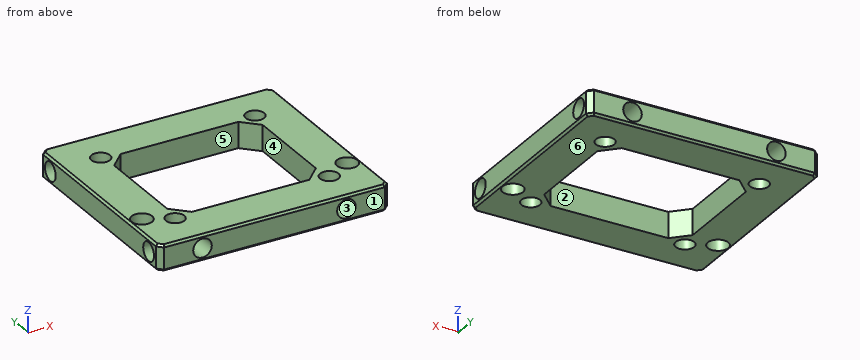
from build123d import *

# Parameters (mm, degrees)
SKETCH2_W               = 44.8
SKETCH2_H               = 39.8
SKETCH2_W_2             = 28.8
SKETCH2_H_2             = 23.8
BOSS_EXTRUDE1_DEPTH     = 5
CHAMFER1_SIZE           = 1
CHAMFER2_SIZE           = 3
SKETCH3_R               = 1.8
CUT_EXTRUDE1_DEPTH      = 6
SKETCH4_R               = 1.8
CUT_EXTRUDE2_DEPTH      = 5
SKETCH5_R               = 1.8
CUT_EXTRUDE3_DEPTH      = 5
MIRROR2_COPY_1_SKETCH_R = 1.8
MIRROR2_COPY_1_DEPTH    = 6
MIRROR2_COPY_2_SKETCH_R = 1.8
MIRROR2_COPY_2_DEPTH    = 5
MIRROR2_COPY_3_SKETCH_R = 1.8
MIRROR2_COPY_3_DEPTH    = 5
SKETCH6_R               = 2
CUT_EXTRUDE4_DEPTH      = 6
CHAMFER3_SIZE           = 0.4


with BuildPart() as part:
    # Sketch2 → Boss-Extrude1 (new body)
    with BuildSketch(Plane.XY):
        Rectangle(SKETCH2_W, SKETCH2_H)
        Rectangle(SKETCH2_W_2, SKETCH2_H_2, mode=Mode.SUBTRACT)
    extrude(amount=BOSS_EXTRUDE1_DEPTH)

    # Chamfer1
    chamfer1_edges = [part.edges().sort_by_distance(p)[0] for p in [
        (-22.4, 19.9, 2.5),
        (22.4, 19.9, 2.5),
        (22.4, -19.9, 2.5),
        (-22.4, -19.9, 2.5),
    ]]
    chamfer(chamfer1_edges, length=CHAMFER1_SIZE)

    # Chamfer2
    chamfer2_edges = [part.edges().sort_by_distance(p)[0] for p in [
        (-14.4, 11.9, 2.5),
        (-14.4, -11.9, 2.5),
        (14.4, -11.9, 2.5),
        (14.4, 11.9, 2.5),
    ]]
    chamfer(chamfer2_edges, length=CHAMFER2_SIZE)

    # Sketch3 → Cut-Extrude1 (cut, through all)
    with BuildSketch(Plane.XY.offset(5)):
        with Locations((14.95, 12.45)):
            Circle(SKETCH3_R)
    cut_extrude1 = extrude(amount=-CUT_EXTRUDE1_DEPTH, mode=Mode.SUBTRACT)

    # Sketch4 → Cut-Extrude2 (cut)
    with BuildSketch(Plane(origin=(0, 19.9, 0), x_dir=(1, 0, 0), z_dir=(0, 1, 0))):
        with Locations((13.95, -2.5)):
            Circle(SKETCH4_R)
    cut_extrude2 = extrude(amount=-CUT_EXTRUDE2_DEPTH, mode=Mode.SUBTRACT)

    # Sketch5 → Cut-Extrude3 (cut)
    with BuildSketch(Plane(origin=(22.4, 0, 0), x_dir=(0, 0, -1), z_dir=(1, 0, 0))):
        with Locations((-2.5, 16.45)):
            Circle(SKETCH5_R)
    cut_extrude3 = extrude(amount=-CUT_EXTRUDE3_DEPTH, mode=Mode.SUBTRACT)

    # Mirror1: Cut-Extrude1, Cut-Extrude2, Cut-Extrude3 across plane
    add(cut_extrude1.mirror(Plane.ZX), mode=Mode.SUBTRACT)
    add(cut_extrude2.mirror(Plane.ZX), mode=Mode.SUBTRACT)
    add(cut_extrude3.mirror(Plane.ZX), mode=Mode.SUBTRACT)

    # Mirror2: Cut-Extrude1, Cut-Extrude2, Cut-Extrude3 across plane
    add(cut_extrude1.mirror(Plane(origin=(0, 0, 0), x_dir=(0, 0, 1), z_dir=(1, 0, 0))), mode=Mode.SUBTRACT)
    add(cut_extrude2.mirror(Plane(origin=(0, 0, 0), x_dir=(0, 0, 1), z_dir=(1, 0, 0))), mode=Mode.SUBTRACT)
    add(cut_extrude3.mirror(Plane(origin=(0, 0, 0), x_dir=(0, 0, 1), z_dir=(1, 0, 0))), mode=Mode.SUBTRACT)

    # Mirror2 copy 1 sketch → Mirror2 copy 1 (cut, through all)
    with BuildSketch(Plane(origin=(0, 0, 5), x_dir=(-1, 0, 0), z_dir=(0, 0, 1))):
        with Locations((14.95, 12.45)):
            Circle(MIRROR2_COPY_1_SKETCH_R)
    extrude(amount=-MIRROR2_COPY_1_DEPTH, mode=Mode.SUBTRACT)

    # Mirror2 copy 2 sketch → Mirror2 copy 2 (cut)
    with BuildSketch(Plane(origin=(0, -19.9, 0), x_dir=(-1, 0, 0), z_dir=(0, -1, 0))):
        with Locations((13.95, -2.5)):
            Circle(MIRROR2_COPY_2_SKETCH_R)
    extrude(amount=-MIRROR2_COPY_2_DEPTH, mode=Mode.SUBTRACT)

    # Mirror2 copy 3 sketch → Mirror2 copy 3 (cut)
    with BuildSketch(Plane(origin=(-22.4, 0, 0), x_dir=(0, 0, -1), z_dir=(-1, 0, 0))):
        with Locations((-2.5, 16.45)):
            Circle(MIRROR2_COPY_3_SKETCH_R)
    extrude(amount=-MIRROR2_COPY_3_DEPTH, mode=Mode.SUBTRACT)

    # Sketch6 → Cut-Extrude4 (cut, through all)
    with BuildSketch(Plane.XY.offset(5)):
        with Locations((19.9, -9.9)):
            Circle(SKETCH6_R)
        with Locations((-19.9, -9.9)):
            Circle(SKETCH6_R)
    extrude(amount=-CUT_EXTRUDE4_DEPTH, mode=Mode.SUBTRACT)

    # Chamfer3
    chamfer3_edges = [part.edges().sort_by_distance(p)[0] for p in [
        (0, -19.9, 0),
        (0, -19.9, 5),
        (-22.4, 0, 0),
        (0, 19.9, 0),
        (22.4, 0, 0),
        (-21.9, 19.4, 0),
        (21.9, 19.4, 0),
        (21.9, -19.4, 0),
        (-21.9, -19.4, 0),
        (-22.4, 0, 5),
        (22.4, 0, 5),
        (0, 19.9, 5),
        (-21.9, 19.4, 5),
        (21.9, 19.4, 5),
        (21.9, -19.4, 5),
        (-21.9, -19.4, 5),
    ]]
    chamfer(chamfer3_edges, length=CHAMFER3_SIZE)


solid = part.part
Geometry check sheet. Reference: the model listing, model coordinates, mm. Face numbers are marked on the shaded views. A direction names the side the tool comes from. Give positions to 0.01 mm unless a question says otherwise; leave off trailing zeros. Write each loop counter-clockwise with the first axis right and the second up, starting at its lowest first coordinate (ties: lowest second). Pieces come first, ordered by that corner, then holes. Notation, with made-up numbers: (-39, 2.25) - (-15, 2.25) arc R8 ccw to (-15, 13.25) - close; hole circle Ø4 at (-16.75, 5.5). An arc over 180 degrees is marked (long way). Put each result on its own line as item: value.
1. Set-up check for the marked faces 5 and 6: record each of +Z, -Z, +X, -X, +Y, -Y from which the full face is reachable in a straight line by a thin tool's end or side.
Ans:
face 5: +Z, -Z
face 6: -Z, +X, -X, +Y, -Y
2. Sectioned sample at C-C, the plane x = -2.5. Enter the section's corners in (y, z).
Ans:
outline: (-19.9, 0.4) - (-19.5, 0) - (-11.9, 0) - (-11.9, 5) - (-19.5, 5) - (-19.9, 4.6) - close; (11.9, 0) - (19.5, 0) - (19.9, 0.4) - (19.9, 4.6) - (19.5, 5) - (11.9, 5) - close
3. Go/stop test with flat-tipped pins: pin 1 (5 mm diameter, centred on x = 3, y = -12, fed in from -Z); pin 2 (1.1 mm diameter, centred on y = 16.5, z = 3, fed in from -X); pin 3 (1.8 mm diameter, centred on y = -16.5, z = 3, fed in from +X); pin 4 (3 mm diameter, centred on x = -13.95, z = 2.5, fed in from -Y). Record where each tip stops, or that it passes through.
Ans:
pin 1: stops at z = 0
pin 2: stops at x = -17.4
pin 3: stops at x = 17.4
pin 4: stops at y = -14.9
4. Sectioned sample at D-D, the plane y = 7. Enter the section's corners in (x, z), plus the area to 3 significant figures.
Ans:
outline: (-22.4, 0.4) - (-22, 0) - (-14.4, 0) - (-14.4, 5) - (-22, 5) - (-22.4, 4.6) - close; (14.4, 0) - (22, 0) - (22.4, 0.4) - (22.4, 4.6) - (22, 5) - (14.4, 5) - close
area: 79.7 mm²
5. Sectioned sample at A-A, the plane x = 19.9. Enter the section's corners in (y, z), plus the area to 3 significant figures.
Ans:
outline: (-19.9, 0.4) - (-19.5, 0) - (-11.9, 0) - (-11.9, 5) - (-19.5, 5) - (-19.9, 4.6) - close; (-7.9, 0) - (19.5, 0) - (19.9, 0.4) - (19.9, 4.6) - (19.5, 5) - (-7.9, 5) - close; hole circle Ø3.6 at (-16.45, 2.5); hole circle Ø3.6 at (16.45, 2.5)
area: 158 mm²
6. Thickness scan on line 1 (X direction, y = -16.8, z = 2.5); line 2 (X direction, y = 18.4, z = 2.5); line 3 (Z direction, x = -13.95, y = -16.45). Record the ranges inside material, lowest first.
Ans:
line 1: x = -17.4 to -15.75, -12.15 to 12.15, 15.75 to 17.4
line 2: x = -22.4 to -15.75, -12.15 to 12.15, 15.75 to 22.4
line 3: z = 0 to 0.7, 4.3 to 5
7. Sectioned sample at B-B, the plane y = -12.45. Enter the section's corners in (x, z), plus the area to 3 significant figures.
Ans:
outline: (-22.4, 0.4) - (-22, 0) - (-16.75, 0) - (-16.75, 5) - (-22, 5) - (-22.4, 4.6) - close; (-13.15, 0) - (13.15, 0) - (13.15, 5) - (-13.15, 5) - close; (16.75, 0) - (22, 0) - (22.4, 0.4) - (22.4, 4.6) - (22, 5) - (16.75, 5) - close
area: 188 mm²
8. Draft check along Y on the marked faces 1, 2, 3 and 4. Enter one of: +Y half, -Y half, draft (parallel to the pull), parting line (faces both ways), or undercut.
Ans:
face 1: -Y half
face 2: undercut
face 3: draft
face 4: undercut
